Could you check a few things on this model? Use its own coordinates, in mm. A direction names the side the tool comes from. Coordinates: 2 decimals unless noted, no trailing zeros. Order: outer loops, then holes, each group sorted by start corner. A loop starts at its lowest first (then second) coordinate and runs counter-clockwise, first axis right, second up. Notation, with made-up numbers: (7, 17) - (50, 17) arc R21 ccw to (50, 51) - close; hole circle Ø1 at (16.5, 65.25). An arc over 180 degrees is marked (long way). Answer as CSV lines item,"result". Start each with the question number.
1. I want a section at C-C, the plane z = 0.5. List the corners of the cut face in (x, y) for me.
2. I want a section at D-D, the plane y = -6.5. List the corners of the cut face in (x, z) for me.
3. For faces 4 (the face through (-10.3, 5.7, -1.5)), 5 (the face through (0, -15, 1)), which set-ups out of +Z, -Z, +X, -X, +Y, -Y let a thin tool reach every point of the face, with its end or its side?
4. I want a section at B-B, the plane x = 0. List the corners of the cut face in (y, z) for me.
5. Thinking about a two-plate mould opening in Y: for faces 1 (the face through (-1, -14, -0.5)), 2 (the face through (3, 0, -2.5)), 3 (the face through (-3.317, -14.936, 0.035)), which applies, released by +Y, released by -Y, zero draft, split by the parting line, or undercut?
6. For pin 1 (1 mm diameter, centred on x = -1.5, z = -1, fed in from -Y); pin 2 (1 mm diameter, centred on x = 7, z = 0.5, fed in from -Y); pin 3 (2 mm diameter, centred on x = 11.5, y = -6, fed in from +Z); pin 4 (3 mm diameter, centred on x = -1, y = -12.5, fed in from +Z), each with a flat end and sliding along its axis, tell me the tip position at first contact or that it passes through.
7. I need wall thicknesses on probe 1 along Y at (x, z) = (0, 0.5); probe 2 along Y at (x, z) = (13, 1.05); probe 3 along X at (y, z) = (7, 0.1). Which ranges of each line are inside material? Lowest first, please.
8. I want a section at A-A, the plane y = 0. List the corners of the cut face in (x, z) for me.
from build123d import *

# Parameters (mm, degrees)
SKETCH_1_R               = 15.3
SKETCH_1_R_2             = 1.1
EXTRUDE_1_DEPTH          = 2.5
SKETCH_2_R               = 1.25
CUT_EXTRUDE_1_DEPTH      = 23.207656337
SKETCH_2_2_R             = 2
CUT_EXTRUDE_2_DEPTH      = 3
PATTERN_CIRCULAR_1_COUNT = 6


with BuildPart() as part:
    # 草图1 → 凸台-拉伸1 (new, symmetric)
    with BuildSketch(Plane.XY):
        Circle(SKETCH_1_R)
        Circle(SKETCH_1_R_2, mode=Mode.SUBTRACT)
    extrude(amount=EXTRUDE_1_DEPTH, both=True)

    # 草图2 → 切除-拉伸1 (cut, through all)
    with BuildSketch(Plane.XY.offset(2.5)):
        with Locations((0, 13)):
            Circle(SKETCH_2_R)
    cut_extrude_1 = extrude(amount=-CUT_EXTRUDE_1_DEPTH, mode=Mode.SUBTRACT)

    # 草图2<2> → 切除-拉伸2 (cut)
    with BuildSketch(Plane.XY.offset(2.5)):
        with Locations((0, 13)):
            Circle(SKETCH_2_2_R)
    cut_extrude_2 = extrude(amount=-CUT_EXTRUDE_2_DEPTH, mode=Mode.SUBTRACT)

    # 阵列(圆周)1: 切除-拉伸1, 切除-拉伸2 ×6 about axis
    pattern_circular_1_axis = Axis((0, 0, 0), (0, 0, 1))
    add([cut_extrude_1.rotate(pattern_circular_1_axis, i * 360 / PATTERN_CIRCULAR_1_COUNT) for i in range(1, PATTERN_CIRCULAR_1_COUNT)], mode=Mode.SUBTRACT)
    add([cut_extrude_2.rotate(pattern_circular_1_axis, i * 360 / PATTERN_CIRCULAR_1_COUNT) for i in range(1, PATTERN_CIRCULAR_1_COUNT)], mode=Mode.SUBTRACT)


solid = part.part
Solved:
1,outline,"circle Ø30.6 at (0, 0); hole circle Ø4 at (-11.26, -6.5); hole circle Ø4 at (-11.26, 6.5); hole circle Ø4 at (0, -13); hole circle Ø4 at (0, 13); hole circle Ø2.2 at (0, 0); hole circle Ø4 at (11.26, -6.5); hole circle Ø4 at (11.26, 6.5)"
2,outline,"(-13.85, -2.5) - (-12.51, -2.5) - (-12.51, -0.5) - (-13.26, -0.5) - (-13.26, 2.5) - (-13.85, 2.5) - close; (-10.01, -2.5) - (10.01, -2.5) - (10.01, -0.5) - (9.26, -0.5) - (9.26, 2.5) - (-9.26, 2.5) - (-9.26, -0.5) - (-10.01, -0.5) - close; (12.51, -2.5) - (13.85, -2.5) - (13.85, 2.5) - (13.26, 2.5) - (13.26, -0.5) - (12.51, -0.5) - close"
3,face 4,"+Z, -Z"
3,face 5,"+Z"
4,outline,"(-15.3, -2.5) - (-14.25, -2.5) - (-14.25, -0.5) - (-15, -0.5) - (-15, 2.5) - (-15.3, 2.5) - close; (-11.75, -2.5) - (-1.1, -2.5) - (-1.1, 2.5) - (-11, 2.5) - (-11, -0.5) - (-11.75, -0.5) - close; (1.1, -2.5) - (11.75, -2.5) - (11.75, -0.5) - (11, -0.5) - (11, 2.5) - (1.1, 2.5) - close; (14.25, -2.5) - (15.3, -2.5) - (15.3, 2.5) - (15, 2.5) - (15, -0.5) - (14.25, -0.5) - close"
5,face 1,"undercut"
5,face 2,"zero draft"
5,face 3,"split by the parting line"
6,pin 1,"stops at y = -15.27"
6,pin 2,"stops at y = -13.85"
6,pin 3,"stops at z = -0.5"
6,pin 4,"stops at z = 2.5"
7,probe 1,"y = -15.3 to -15, -11 to -1.1, 1.1 to 11, 15 to 15.3"
7,probe 2,"y = -8.07 to -7.48, -5.52 to 5.52, 7.48 to 8.07"
7,probe 3,"x = -13.6 to -13.19, -9.32 to 9.32, 13.19 to 13.6"
8,outline,"(-15.3, -2.5) - (-1.1, -2.5) - (-1.1, 2.5) - (-15.3, 2.5) - close; (1.1, -2.5) - (15.3, -2.5) - (15.3, 2.5) - (1.1, 2.5) - close"
